Autodesk Inventor part; units mm, degrees
ref_plane "YZ Plane" through (0, 0, 0) normal (1, 0, 0) x (0, 1, 0)
ref_plane "XZ Plane" through (0, 0, 0) normal (0, 1, 0) x (-1, 0, 0)
ref_plane "XY Plane" through (0, 0, 0) normal (0, 0, 1) x (1, 0, 0)
sketch "스케치3" plane through (0, 0, 0) normal (0, 1, 0) x (-1, 0, 0)
  line L0 (68.1838, -28.2426) -> (28.2426, -68.1838)
  line L1 (28.2426, -68.1838) -> (-28.2426, -68.1838)
  line L2 (-28.2426, -68.1838) -> (-68.1838, -28.2426)
  line L3 (-68.1838, -28.2426) -> (-68.1838, 28.2426)
  line L4 (-68.1838, 28.2426) -> (-28.2426, 68.1838)
  line L5 (-28.2426, 68.1838) -> (28.2426, 68.1838)
  line L6 (28.2426, 68.1838) -> (68.1838, 28.2426)
  line L7 (68.1838, 28.2426) -> (68.1838, -28.2426)
  line L8 (65.1838, -27) -> (27, -65.1838)
  line L9 (27, -65.1838) -> (-27, -65.1838)
  line L10 (-27, -65.1838) -> (-65.1838, -27)
  line L11 (-65.1838, -27) -> (-65.1838, 27)
  line L12 (-65.1838, 27) -> (-27, 65.1838)
  line L13 (-27, 65.1838) -> (27, 65.1838)
  line L14 (27, 65.1838) -> (65.1838, 27)
  line L15 (65.1838, 27) -> (65.1838, -27)
  point P0 (0, 0)
  point P1 (0, 0)
  point P2 (0, 0)
  point P3 (0, 0)
  dimension "d43" = 54
  dimension "d44" = 3
extrude "돌출2" add sketch "스케치3" along normal blind 6.8 contours L0 L1 L2 L3 L4 L5 L6 L7 | L8 L9 L10 L11 L12 L13 L14 L15
sketch "스케치4" plane through (0, 6.8, 0) normal (0, 1, 0) x (1, 0, 0)
  line L0 (26.8343, -64.7838) -> (-26.8343, -64.7838)
  line L1 (-26.8343, -64.7838) -> (-64.7838, -26.8343)
  line L2 (-64.7838, -26.8343) -> (-64.7838, 26.8343)
  line L3 (-64.7838, 26.8343) -> (-26.8343, 64.7838)
  line L4 (-26.8343, 64.7838) -> (26.8343, 64.7838)
  line L5 (26.8343, 64.7838) -> (64.7838, 26.8343)
  line L6 (64.7838, 26.8343) -> (64.7838, -26.8343)
  line L7 (64.7838, -26.8343) -> (26.8343, -64.7838)
  line L8 (-27.5799, 66.5838) -> (27.5799, 66.5838)
  line L9 (27.5799, 66.5838) -> (66.5838, 27.5799)
  line L10 (66.5838, 27.5799) -> (66.5838, -27.5799)
  line L11 (66.5838, -27.5799) -> (27.5799, -66.5838)
  line L12 (27.5799, -66.5838) -> (-27.5799, -66.5838)
  line L13 (-27.5799, -66.5838) -> (-66.5838, -27.5799)
  line L14 (-66.5838, -27.5799) -> (-66.5838, 27.5799)
  line L15 (-66.5838, 27.5799) -> (-27.5799, 66.5838)
  line L16 (-26.7515, 64.5838) -> (26.7515, 64.5838)
  line L17 (26.7515, 64.5838) -> (64.5838, 26.7515)
  line L18 (64.5838, 26.7515) -> (64.5838, -26.7515)
  line L19 (64.5838, -26.7515) -> (26.7515, -64.5838)
  line L20 (26.7515, -64.5838) -> (-26.7515, -64.5838)
  line L21 (-26.7515, -64.5838) -> (-64.5838, -26.7515)
  line L22 (-64.5838, -26.7515) -> (-64.5838, 26.7515)
  line L23 (-64.5838, 26.7515) -> (-26.7515, 64.5838)
  line L24 (-68.1838, 28.2426) -> (-68.1838, -28.2426)
  point P0 (0, 0)
  point P1 (0, 0)
  point P2 (0, 0)
  point P3 (0, 0)
  dimension "d42" = 1.8
  dimension "d45" = 0.2
  dimension "d60" = 1.6
extrude "돌출3" cut sketch "스케치4" against normal blind 2 contours L0 L1 L2 L3 L4 L5 L6 L7 | L8 L9 L10 L11 L12 L13 L14 L15 | L16 L17 L18 L19 L20 L21 L22 L23
sketch "스케치5" plane through (0, 0, 0) normal (0, -1, 0) x (1, 0, 0)
  line L0 (10, 2.5) -> (20, 2.5)
  line L1 (20, 2.5) -> (20, -2.5)
  line L2 (20, -2.5) -> (10, -2.5)
  line L3 (10, -2.5) -> (10, 2.5)
  line L4 (10, 2.5) -> (20, -2.5) construction
  line L5 (20, 2.5) -> (10, -2.5) construction
  line L6 (-20, 2.5) -> (-10, 2.5)
  line L7 (-10, 2.5) -> (-10, -2.5)
  line L8 (-10, -2.5) -> (-20, -2.5)
  line L9 (-20, -2.5) -> (-20, 2.5)
  line L10 (-20, 2.5) -> (-10, -2.5) construction
  line L11 (-10, 2.5) -> (-20, -2.5) construction
  point P0 (0, 0)
  point P1 (15, 0)
  point P2 (-15, 0)
  dimension "d11" = 10
  dimension "d12" = 5
  dimension "d13" = 10
  dimension "d16" = 30
extrude "돌출4" add sketch "스케치5" along normal blind 10
sketch "스케치6" plane through (-10, 0, -2.5) normal (0, 0, -1) x (-1, 0, 0)
  circle A0 centre (5, -10) radius 5
  circle A1 centre (-25, -10) radius 5
  line L0 (-20, -10) -> (-30, -10)
  line L1 (10, -10) -> (0, -10)
  point P0 (-10, 0)
  dimension "d23" = 10
  dimension "d24" = 10
extrude "돌출5" add sketch "스케치6" against normal blind 5
sketch "스케치7" plane through (-10, 0, -2.5) normal (0, 0, -1) x (-1, 0, 0)
  circle A0 centre (5, -10) radius 1.25
  line L0 (10, 0) -> (10, -10)
  line L1 (0, 0) -> (10, 0)
  line L2 (4.7788, 0) -> (0, 0)
  circle A1 centre (-25, -10) radius 1.25
  point P0 (-10, 0)
  dimension "d27" = 2.5
  dimension "d28" = 5
  dimension "d31" = 30
extrude "돌출6" cut sketch "스케치7" against normal blind 5
sketch "스케치8" plane through (0, 0, 0) normal (0, -1, 0) x (1, 0, 0)
  circle A0 centre (0, -35) radius 1.25
  line L0 (-10, 2.5) -> (-10, -2.5)
  point P0 (0, 0)
  point P1 (-10, 0)
  dimension "d38" = 2.5
  dimension "d39" = 35
sketch "스케치9" plane through (0, 4.8, 0) normal (0, 1, 0) x (1, 0, 0)
  line L0 (-26.7515, 64.5838) -> (26.7515, 64.5838)
  line L1 (26.7515, 64.5838) -> (64.5838, 26.7515)
  line L2 (64.5838, 26.7515) -> (64.5838, -26.7515)
  line L3 (64.5838, -26.7515) -> (26.7515, -64.5838)
  line L4 (26.7515, -64.5838) -> (-26.7515, -64.5838)
  line L5 (-26.7515, -64.5838) -> (-64.5838, -26.7515)
  line L6 (-64.5838, -26.7515) -> (-64.5838, 26.7515)
  line L7 (-64.5838, 26.7515) -> (-26.7515, 64.5838)
  line L8 (-27.5799, 66.5838) -> (27.5799, 66.5838)
  line L9 (-25.5088, 61.5838) -> (25.5088, 61.5838)
  line L10 (25.5088, 61.5838) -> (61.5838, 25.5088)
  line L11 (61.5838, 25.5088) -> (61.5838, -25.5088)
  line L12 (61.5838, -25.5088) -> (25.5088, -61.5838)
  line L13 (25.5088, -61.5838) -> (-25.5088, -61.5838)
  line L14 (-25.5088, -61.5838) -> (-61.5838, -25.5088)
  line L15 (-61.5838, -25.5088) -> (-61.5838, 25.5088)
  line L16 (-61.5838, 25.5088) -> (-25.5088, 61.5838)
  point P0 (0, 0)
  point P1 (0, 0)
  point P2 (0, 0)
  dimension "d46" = 2
  dimension "d47" = 3
extrude "돌출8" add sketch "스케치9" along normal blind 0.8 contours L0 L1 L2 L3 L4 L5 L6 L7 | L9 L10 L11 L12 L13 L14 L15 L16
fillet "모깎기1" radius 1.2 16 edges at (-68.1838, 6.8, 0) (-48.2132, 6.8, 48.2132) (0, 6.8, 68.1838) (48.2132, 6.8, 48.2132) (68.1838, 6.8, 0) (48.2132, 6.8, -48.2132) (0, 6.8, -68.1838) (-48.2132, 6.8, -48.2132) (48.2132, 0, 48.2132) (0, 0, 68.1838) (-48.2132, 0, 48.2132) (-68.1838, 0, 0) (-48.2132, 0, -48.2132) (0, 0, -68.1838) (48.2132, 0, -48.2132) (68.1838, 0, 0)
sketch "스케치10" plane through (0, 0, 0) normal (0, -1, 0) x (1, 0, 0)
  line L0 (-20, 2.5) -> (-10, 2.5)
  line L1 (-10, -2.5) -> (-20, -2.5)
  line L2 (-20, 2.5) -> (-19, 2.5)
  line L3 (-19, 2.5) -> (-19, -2.5)
  line L4 (-19, -2.5) -> (-20, -2.5)
  line L5 (-20, -2.5) -> (-20, 2.5)
  line L6 (20, -2.5) -> (10, -2.5)
  line L7 (10, 2.5) -> (20, 2.5)
  line L8 (20, -2.5) -> (19, -2.5)
  line L9 (19, -2.5) -> (19, 2.5)
  line L10 (19, 2.5) -> (20, 2.5)
  line L11 (20, 2.5) -> (20, -2.5)
  point P0 (0, 0)
  dimension "d54" = 1
  dimension "d55" = 1
extrude "돌출9" cut sketch "스케치10" along normal blind 15
extrude "돌출10" cut sketch "스케치8" against normal up to surface (5.6 mm away)
equation "\"d55\" = d54"
properties part number "OV-PAM_top_2"
Model file for the job. Use its own axes, mm. A direction names the side the tool comes from. Coordinates: 2 decimals unless noted, no trailing zeros. Write each loop counter-clockwise with the first axis right and the second up, starting at its lowest first coordinate (ties: lowest second). Pieces come first, ordered by that corner, then holes. Notation, with made-up numbers: (36, 76.5) - (53, 76.5) arc R22 cw to (53, 97.5) - close; hole circle Ø4 at (15, -35). An arc over 180 degrees is marked (long way). One line per item, written item: value. Start each with the question number.
1. Tool access for faces 4 (the flat face through (-15, -7, 2.5)), 5 (the flat face through (19, -6, 0)), 6 (the flat face through (-10, -5, 0)): list every direction of +Z, -Z, +X, -X, +Y, -Y with a clear straight run to the whole face (end or side of a thin tool).
2. Mould opens along Z. For faces 1 (the cylindrical face through (-13.336, -14.715, -0.035)), 2 (the cylindrical face through (-48.238, 0.342, 47.678)), 3 (the flat face through (47.355, 5.814, 46.809)) say: released by +Z, released by -Z, zero draft, split by the parting line, or undercut.
3. Probe line 1 (Y direction, x = -15, z = 1.05); line 2 (Z direction, x = 0, y = 4.45); line 3 (X direction, y = -7, z = -1). List the from-to ranges inside material, lowest first. Write a range as from..to.
4. Flat gauge pins, fed straight in: pin 1 (1.5 mm diameter, centred on y = -5.5, z = 1, fed in from -X); pin 2 (0.6 mm diameter, centred on y = 6, z = -0.5, fed in from -X); pin 3 (1.5 mm diameter, centred on x = 15, y = -10, fed in from +Z); pin 4 (2.5 mm diameter, centred on y = -3, z = -1, fed in from +X). Where does each tip first touch, or does it go through?
5. Slice it at A-A (z = 9). Write the cut outline in (x, y).
Answers below:
1. face 4: +Z, +X, -X, -Y
1. face 5: +Z, -Z, +X, -Y
1. face 6: +Z, -Z, -Y
2. face 1: zero draft
2. face 2: released by +Z
2. face 3: undercut
3. line 1: y = -15..-11.25, -8.75..5.6
3. line 2: z = -68.18..-36.25, -33.75..68.18
3. line 3: x = -19..-10, 10..19
4. pin 1: stops at x = -19
4. pin 2: stops at x = -68.18
4. pin 3: passes through
4. pin 4: stops at x = 19
5. outline: (-68.18, 1.2) arc R1.2 ccw to (-66.98, 0) - (66.98, 0) arc R1.2 ccw to (68.18, 1.2) - (68.18, 5.6) arc R1.2 ccw to (66.98, 6.8) - (66.58, 6.8) - (66.58, 4.8) - (64.58, 4.8) - (64.58, 5.6) - (-64.58, 5.6) - (-64.58, 4.8) - (-66.58, 4.8) - (-66.58, 6.8) - (-66.98, 6.8) arc R1.2 ccw to (-68.18, 5.6) - close
